CAD build for the part. Positions are in the model's coordinates, mm. Face numbers are marked on the shaded views. A direction names the side the tool comes from. Round coordinates to 2 decimals unless told otherwise and drop trailing zeros. Write each loop counter-clockwise with the first axis right and the second up, starting at its lowest first coordinate (ties: lowest second). Pieces come first, ordered by that corner, then holes. Notation, with made-up numbers: (49, -12.5) - (92, -12.5) arc R16 ccw to (92, -0.5) - close; hole circle Ø5 at (39, -17). An arc over 180 degrees is marked (long way). Put each result on its own line as item: value. Start each with the question number.
Item 1: Cut at A-A (x = 31.5). Give the cut face in (y, z).
Item 2: Drill centre lines: line 1 (X direction, y = -18.5, z = 1.5); line 2 (X direction, y = -10, z = -14); line 3 (Z direction, x = 29, y = -8). Where is each one in solid material? Low to high. Write a range as from..to.
Item 3: Cut at D-D (y = -5.25). Give the cut face in (x, z).
Item 4: Pin check, flat tips, straight feed: pin 1 Ø2 at (x, y) = (-27.5, -5) entering from +Z; pin 2 Ø5 at (x, y) = (29.5, -13.5) entering from +Z; pin 3 Ø1.6 at (x, y) = (-36.5, -15) entering from +Z. Stop position of each tip, or through.
Item 5: Cut at C-C (y = -10). Give the cut face in (x, z), and give its area (3 significant figures).
Item 6: Mould opens along X. For the marked faces 1, 2 and 3 say: released by +X, released by -X, zero draft, split by the parting line, or undercut.
Item 7: Cut at B-B (z = 25). Give the cut face in (x, y).
Item 8: 3-axis set-ups, long thin cutter, end or side, ignore diameter. For the marked faces 4, 5 and 6: which of +Z, -Z, +X, -X, +Y, -Y reach the whole face in a straight line?
```python
from build123d import *

# Parameters (mm, degrees)
F1_DEPTH = 20
F2_R     = 6
F3_DEPTH = 80.001


with BuildPart() as f1:
    # F0 (on Front) → F1 (new body)
    with BuildSketch(Plane.XZ):
        with BuildLine():
            Line((-34.949345, 11.64024), (-37.002013, 11.64024))
            Line((-37.002013, 11.64024), (-37.002013, -24.35976))
            Line((-37.002013, -24.35976), (-21.002013, -24.35976))
            Line((-21.002013, -24.35976), (-21.002013, -12.35976))
            Line((-21.002013, -12.35976), (-27.002013, -12.35976))
            Line((-27.002013, -12.35976), (-27.002013, 11.64024))
            Line((-27.002013, 11.64024), (-21.002013, 11.64024))
            ThreePointArc((-21.002013, 11.64024), (2.997987, 35.64024), (26.997987, 11.64024))
            Line((26.997987, 11.64024), (32.997987, 11.64024))
            Line((32.997987, 11.64024), (32.997987, -12.35976))
            Line((32.997987, -12.35976), (26.997987, -12.35976))
            Line((26.997987, -12.35976), (26.997987, -24.35976))
            Line((26.997987, -24.35976), (42.997987, -24.35976))
            Line((42.997987, -24.35976), (42.997987, 16.615835))
            Line((42.997987, 16.615835), (40.352251, 16.615835))
            ThreePointArc((40.352251, 16.615835), (39.074416, 17.077285), (38.386237, 18.248699))
            ThreePointArc((38.386237, 18.248699), (29.686172, 35.800968), (13.083165, 46.198729))
            ThreePointArc((13.083165, 46.198729), (11.003561, 47.638801), (10.203741, 50.038561))
            Line((10.203741, 50.038561), (10.203741, 55.64024))
            Line((10.203741, 55.64024), (-4.950045, 55.64024))
            Line((-4.950045, 55.64024), (-4.950045, 49.814112))
            ThreePointArc((-4.950045, 49.814112), (-5.726754, 47.445485), (-7.755242, 45.996725))
            ThreePointArc((-7.755242, 45.996725), (-25.440396, 33.71417), (-32.952117, 13.534977))
            ThreePointArc((-32.952117, 13.534977), (-33.572851, 12.189288), (-34.949345, 11.64024))
        make_face()
    extrude(amount=F1_DEPTH)

    # F2 (on face) → F3 (cut, through all)
    with BuildSketch(Plane.XY.offset(55.64024)):
        with Locations((2.626848, -10)):
            Circle(F2_R)
    extrude(amount=-F3_DEPTH, mode=Mode.SUBTRACT)


solid = f1.part
```
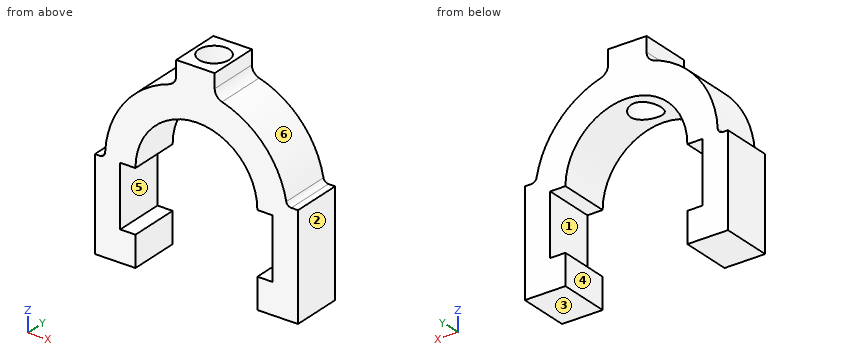
Output values:
1. outline: (-20, -24.36) - (0, -24.36) - (0, -12.36) - (-20, -12.36) - close; (-20, 11.64) - (0, 11.64) - (0, 33.63) - (-20, 33.63) - close
2. line 1: -37..-27, 33..43
2. line 2: -37..-21, 27..43
2. line 3: -24.36..-12.36, 11.64..36.54
3. outline: (-37, -24.36) - (-21, -24.36) - (-21, -12.36) - (-27, -12.36) - (-27, 11.64) - (-21, 11.64) arc R24 cw to (-1.04, 35.3) - (-1.04, 55.64) - (-4.95, 55.64) - (-4.95, 49.81) arc R4 cw to (-7.76, 46) arc R36 ccw to (-32.95, 13.53) arc R2 cw to (-34.95, 11.64) - (-37, 11.64) - close; (6.29, 35.41) arc R24 cw to (27, 11.64) - (33, 11.64) - (33, -12.36) - (27, -12.36) - (27, -24.36) - (43, -24.36) - (43, 16.62) - (40.35, 16.62) arc R2 cw to (38.39, 18.25) arc R36 ccw to (13.08, 46.2) arc R4 cw to (10.2, 50.04) - (10.2, 55.64) - (6.29, 55.64) - close
4. pin 1: z = 32.28
4. pin 2: z = 38.47
4. pin 3: z = 11.64
5. outline: (-37, -24.36) - (-21, -24.36) - (-21, -12.36) - (-27, -12.36) - (-27, 11.64) - (-21, 11.64) arc R24 cw to (-3.37, 34.78) - (-3.37, 55.64) - (-4.95, 55.64) - (-4.95, 49.81) arc R4 cw to (-7.76, 46) arc R36 ccw to (-32.95, 13.53) arc R2 cw to (-34.95, 11.64) - (-37, 11.64) - close; (8.63, 34.97) arc R24 cw to (27, 11.64) - (33, 11.64) - (33, -12.36) - (27, -12.36) - (27, -24.36) - (43, -24.36) - (43, 16.62) - (40.35, 16.62) arc R2 cw to (38.39, 18.25) arc R36 ccw to (13.08, 46.2) arc R4 cw to (10.2, 50.04) - (10.2, 55.64) - (8.63, 55.64) - close
5. area: 1,900 mm2
6. face 1: undercut
6. face 2: released by +X
6. face 3: zero draft
7. outline: (-30.43, -20) - (-16.94, -20) - (-16.94, 0) - (-30.43, 0) - close; (22.94, -20) - (36.43, -20) - (36.43, 0) - (22.94, 0) - close
8. face 4: -Z, +Y, -Y
8. face 5: +Y, -Y
8. face 6: +Z, +X, +Y, -Y
